Check sheet for the modelled part. Datum: model origin and axes. Units: mm. Face numbers are marked on the shaded views. A direction names the side the tool comes from. Round coordinates to 2 decimals unless told otherwise and drop trailing zeros. Order: outer loops, then holes, each group sorted by start corner. A loop starts at its lowest first (then second) coordinate and runs counter-clockwise, first axis right, second up.
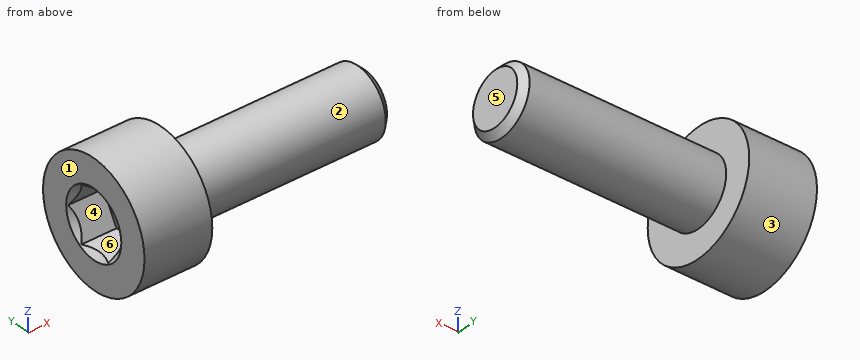
```python
from build123d import *

# Parameters (mm, degrees)
SKETCH2_R           = 1.5
BOSS_EXTRUDE1_DEPTH = 9
CHAMFER1_SIZE       = 0.3
SKETCH6_W           = 3
SKETCH6_H           = 2.75
CUT_EXTRUDE1_DEPTH  = 1.6
SKETCH8_R           = 1.493375673
CUT_EXTRUDE2_DEPTH  = 1
CUT_EXTRUDE2_DRAFT  = -45


with BuildPart() as part:
    # Sketch2 → Boss-Extrude1 (new body)
    with BuildSketch(Plane(origin=(0, 0, 0), x_dir=(0, 0, -1), z_dir=(1, 0, 0))):
        Circle(SKETCH2_R)
    extrude(amount=-BOSS_EXTRUDE1_DEPTH)

    # Chamfer1
    chamfer1_edges = [part.edges().sort_by_distance(p)[0] for p in [
        (0, 0, 1.5),
    ]]
    chamfer(chamfer1_edges, length=CHAMFER1_SIZE)

    # Sketch6 → Revolve1 (revolve)
    with BuildSketch(Plane.XY):
        with Locations((-10.5, 1.375)):
            Rectangle(SKETCH6_W, SKETCH6_H)
    revolve(axis=Axis((-9, 0, 0), (-1, 0, 0)))

    # Sketch7 → Cut-Extrude1 (cut)
    with BuildSketch(Plane.ZY.offset(12)):
        Polygon((0, 1.443375673), (-1.25, 0.721687836), (-1.25, -0.721687836), (0, -1.443375673), (1.25, -0.721687836), (1.25, 0.721687836), align=None)
    extrude(amount=-CUT_EXTRUDE1_DEPTH, mode=Mode.SUBTRACT)


with BuildPart() as cut_extrude2_tool:
    # Sketch8 → Cut-Extrude2 (with draft: the straight prism first)
    with BuildSketch(Plane.ZY.offset(12)):
        Circle(SKETCH8_R)
    extrude(amount=-CUT_EXTRUDE2_DEPTH)
    # Cut-Extrude2: the draft: its side faces are tilted about the plane it starts from
    cut_extrude2_sides = [cut_extrude2_tool.faces().sort_by_distance(p)[0] for p in [
        (-11.5, 0, -1.493375673),
    ]]
    draft(cut_extrude2_sides, Plane.ZY.offset(12), CUT_EXTRUDE2_DRAFT)


with BuildPart() as part_1:
    add(part.part)

    # Cut-Extrude2: cut by cut_extrude2_tool
    add(cut_extrude2_tool.part, mode=Mode.SUBTRACT)


solid = part_1.part
```
Item 1: Sectioned sample at A-A (y = 0). Record the cut outline in (x, z).
Answer:
outline: (-12, -2.75) - (-9, -2.75) - (-9, -1.5) - (-0.3, -1.5) - (0, -1.2) - (0, 1.2) - (-0.3, 1.5) - (-9, 1.5) - (-9, 2.75) - (-12, 2.75) - (-12, 1.49) - (-11.76, 1.25) - (-10.4, 1.25) - (-10.4, -1.25) - (-11.76, -1.25) - (-12, -1.49) - close
Item 2: Sectioned sample at C-C (z = -1.8). Record the cut outline in (x, y), and give its area (3 significant figures).
Answer:
outline: (-12, -2.08) - (-9, -2.08) - (-9, 2.08) - (-12, 2.08) - close
area: 12.5 mm2
Item 3: Access from +Z, -Z, +X, -X, +Y, -Y to the whole of each face (thin tool, end or side, straight path). Record for the marked faces 1 and 2.
Answer:
face 1: +Z, -Z, -X, +Y, -Y
face 2: +X
Item 4: Release check for a two-part mould opening along Y. For the marked faces 3, 4, 5 and 6 record: released by +Y, released by -Y, zero draft, split by the parting line, or undercut.
Answer:
face 3: split by the parting line
face 4: undercut
face 5: zero draft
face 6: undercut
Item 5: Scan lines: line 1 along Z through (x, y) = (-3, -0.9); line 2 along Y through (x, z) = (-1.5, 0.4); line 3 along X through (y, z) = (0.65, -0.05). Record each from-to range of solid material in increasing order.
Answer:
line 1: z = -1.2 to 1.2
line 2: y = -1.45 to 1.45
line 3: x = -10.4 to 0
Item 6: Go/stop test with flat-tipped pins: P1, Ø3, axis at x = -8, y = 1.5, coming from the -Z side; P2, Ø0.8, axis at y = 0, z = -0.5, coming from the -X side. Record where each tip stops, or that it passes through.
Answer:
P1: stops at z = -2.72
P2: stops at x = -10.4
Item 7: Sectioned sample at D-D (z = 2.45). Record the cut outline in (x, y).
Answer:
outline: (-12, -1.25) - (-9, -1.25) - (-9, 1.25) - (-12, 1.25) - close
Item 8: Sectioned sample at B-B (x = -2). Record the cut outline in (y, z).
Answer:
outline: circle Ø3 at (0, 0)
